```python
from build123d import *

# Parameters (mm, degrees)
F0_W         = 80
F0_H         = 80
F1_DEPTH     = 30
F2_W         = 60
F2_H         = 25
F3_DEPTH     = 10
F4_W         = 60
F4_H         = 25
F5_DEPTH     = 10
F6_R         = 5
F7_DEPTH     = 100.001
F8_W         = 50
F8_H         = 40
F9_DEPTH     = 30.001
F10_R        = 6.35
F11_T1_DEPTH = 41.75
F11_T3_DEPTH = 41.75


# Not quite as in the source:
# - a fillet or chamfer that OpenCascade refuses, or shapes differently, is made with other operations: its cross-section is extruded or revolved along the edge and cut away or added


with BuildPart() as f1:
    # F0 (on Top) → F1 (new body)
    with BuildSketch(Plane.XY):
        Rectangle(F0_W, F0_H)
    extrude(amount=F1_DEPTH)

    # F2 (on face) → F3 (join)
    with BuildSketch(Plane(origin=(-40, 0, 0), x_dir=(0, -1, 0), z_dir=(-1, 0, 0))):
        with Locations((0, 15)):
            Rectangle(F2_W, F2_H)
    extrude(amount=F3_DEPTH)

    # F4 (on face) → F5 (join)
    with BuildSketch(Plane.YZ.offset(40)):
        with Locations((0, 15)):
            Rectangle(F4_W, F4_H)
    extrude(amount=F5_DEPTH)

    # F6 (on face) → F7 (cut, through all)
    with BuildSketch(Plane(origin=(-50, 0, 0), x_dir=(0, -1, 0), z_dir=(-1, 0, 0))):
        with Locations((0, 15)):
            Circle(F6_R)
    extrude(amount=-F7_DEPTH, mode=Mode.SUBTRACT)

    # F8 (on face) → F9 (cut, through all)
    with BuildSketch(Plane.XY.offset(30)):
        Rectangle(F8_W, F8_H)
    extrude(amount=-F9_DEPTH, mode=Mode.SUBTRACT)

    # F10
    f10_edges = [f1.edges().sort_by_distance(p)[0] for p in [
        (-25, 20, 15),
        (25, 20, 15),
        (25, -20, 15),
        (-25, -20, 15),
    ]]
    fillet(f10_edges, radius=F10_R)

    # F11: fillet of radius 12.7 on 8 edges, made by hand

    # F11_s2 → F11_t1 (cut)
    with BuildSketch(Plane.YZ.offset(40)):
        with BuildLine():
            ThreePointArc((-30, 14.8), (-26.2802561211, 23.7802561211), (-17.3, 27.5))
            Line((-17.3, 27.5), (-30, 27.5))
            Line((-30, 27.5), (-30, 14.8))
        make_face()
        with BuildLine():
            ThreePointArc((-30, 15.2), (-26.2802561211, 6.2197438789), (-17.3, 2.5))
            Line((-17.3, 2.5), (-30, 2.5))
            Line((-30, 2.5), (-30, 15.2))
        make_face()
        with BuildLine():
            ThreePointArc((30, 15.2), (26.2802561211, 6.2197438789), (17.3, 2.5))
            Line((17.3, 2.5), (30, 2.5))
            Line((30, 2.5), (30, 15.2))
        make_face()
        with BuildLine():
            ThreePointArc((17.3, 27.5), (26.2802561211, 23.7802561211), (30, 14.8))
            Line((30, 14.8), (30, 27.5))
            Line((30, 27.5), (17.3, 27.5))
        make_face()
    extrude(amount=F11_T1_DEPTH, mode=Mode.SUBTRACT)

    # F11_s4 → F11_t3 (cut)
    with BuildSketch(Plane.YZ.offset(-81.75)):
        with BuildLine():
            ThreePointArc((17.3, 2.5), (26.2802561211, 6.2197438789), (30, 15.2))
            Line((30, 15.2), (30, 2.5))
            Line((30, 2.5), (17.3, 2.5))
        make_face()
        with BuildLine():
            ThreePointArc((-17.3, 2.5), (-26.2802561211, 6.2197438789), (-30, 15.2))
            Line((-30, 15.2), (-30, 2.5))
            Line((-30, 2.5), (-17.3, 2.5))
        make_face()
        with BuildLine():
            ThreePointArc((-17.3, 27.5), (-26.2802561211, 23.7802561211), (-30, 14.8))
            Line((-30, 14.8), (-30, 27.5))
            Line((-30, 27.5), (-17.3, 27.5))
        make_face()
        with BuildLine():
            ThreePointArc((30, 14.8), (26.2802561211, 23.7802561211), (17.3, 27.5))
            Line((17.3, 27.5), (30, 27.5))
            Line((30, 27.5), (30, 14.8))
        make_face()
    extrude(amount=F11_T3_DEPTH, mode=Mode.SUBTRACT)


solid = f1.part
```
Check sheet for the modelled part. Datum: model origin and axes. Units: mm. A direction names the side the tool comes from. Coordinates: 2 decimals unless noted, no trailing zeros. Write each loop counter-clockwise with the first axis right and the second up, starting at its lowest first coordinate (ties: lowest second). Pieces come first, ordered by that corner, then holes. Notation, with made-up numbers: M 42.25,89.25 L 92.25,89.25 A16 cw 92.25,111.25 Z; hole C -32,88.25 d9. An arc over 180 degrees is marked long. Use one line per item in the form item = value.
Item 1: Set-up check for faces 4 (the face through (-45, 0, 27.5)), 5 (the face through (-45.07, 26.31, 23.75)), 6 (the face through (-45.07, 26.11, 6.05)), 7 (the face through (0, -20, 15)): record each of +Z, -Z, +X, -X, +Y, -Y from which the full face is reachable in a straight line by a thin tool's end or side.
Answer below:
face_4 = +Z, -X, +Y, -Y
face_5 = +Z, -X, +Y
face_6 = -Z, -X, +Y
face_7 = +Z, -Z
Item 2: Sectioned sample at A-A, the plane y = 0. Record the cut outline in (x, z).
Answer below:
outline = M -50,2.5 L -40,2.5 L -40,0 L -25,0 L -25,10 L -50,10 Z; M -50,20 L -25,20 L -25,30 L -40,30 L -40,27.5 L -50,27.5 Z; M 25,0 L 40,0 L 40,2.5 L 50,2.5 L 50,10 L 25,10 Z; M 25,20 L 50,20 L 50,27.5 L 40,27.5 L 40,30 L 25,30 Z
Item 3: Release check for a two-part mould opening along X. For faces 1 (the face through (-45.07, -26.11, 23.95)), 2 (the face through (23.19, 18.09, 14.79)), 3 (the face through (-50, 0, 21)) record: pulls with the +X half, pulls with the -X half, needs draft (parallel to the pull), parting line crosses it, or undercut.
Answer below:
face_1 = needs draft
face_2 = undercut
face_3 = pulls with the -X half
Item 4: Material ranges on L1, parallel to Y at x = -2, z = 3; L2, parallel to Z at x = -31.5, y = 0; L3, parallel to Z at x = -44.5, y = -0.5, recorded low to high. Write a range as from..to.
Answer below:
L1 = -40..-20, 20..40
L2 = 0..10, 20..30
L3 = 2.5..10.03, 19.97..27.5
Item 5: Gauge pin test, flat ends, axial feed: pin 1 Ø3 at (x, y) = (-44.5, 2.5) entering from -Z; pin 2 Ø5 at (x, y) = (-45, 6.5) entering from +Z. Record the tip position at first contact, or that the pin passes through.
Answer below:
pin_1 = 2.5
pin_2 = 27.5
Item 6: Sectioned sample at C-C, the plane z = 22.25. Record the cut outline in (x, y).
Answer below:
outline = M -50,-27.59 L -40,-27.59 L -40,-40 L 40,-40 L 40,-27.59 L 50,-27.59 L 50,27.59 L 40,27.59 L 40,40 L -40,40 L -40,27.59 L -50,27.59 Z; hole M -25,-13.65 A6.35 ccw -18.65,-20 L 18.65,-20 A6.35 ccw 25,-13.65 L 25,13.65 A6.35 ccw 18.65,20 L -18.65,20 A6.35 ccw -25,13.65 Z
Item 7: Sectioned sample at B-B, the plane x = 12.5. Record the cut outline in (y, z), and give its area (3 significant figures).
Answer below:
outline = M -40,0 L -20,0 L -20,30 L -40,30 Z; M 20,0 L 40,0 L 40,30 L 20,30 Z
area = 1,200 mm^2
Item 8: Sectioned sample at D-D, the plane z = 12.5. Record the cut outline in (x, y), and give its area (3 significant figures).
Answer below:
outline = M -50,-29.71 L -40,-29.71 L -40,-40 L 40,-40 L 40,-29.71 L 50,-29.71 L 50,-4.33 L 25,-4.33 L 25,-13.65 A6.35 cw 18.65,-20 L -18.65,-20 A6.35 cw -25,-13.65 L -25,-4.33 L -50,-4.33 Z; M -50,4.33 L -25,4.33 L -25,13.65 A6.35 cw -18.65,20 L 18.65,20 A6.35 cw 25,13.65 L 25,4.33 L 50,4.33 L 50,29.71 L 40,29.71 L 40,40 L -40,40 L -40,29.71 L -50,29.71 Z
area = 5,190 mm^2
